Read the model definition and answer for the solid it produces. Units are mm, in the model's axes. A direction names the side the tool comes from. Give positions to 0.01 mm unless a question says otherwise; leave off trailing zeros. Write each loop counter-clockwise with the first axis right and the second up, starting at its lowest first coordinate (ties: lowest second). Pieces come first, ordered by that corner, then holes. Notation, with made-up numbers: M 63.25,-13 L 117.25,-13 A28 ccw 117.25,11 Z; hole C 72,28.5 d9. An arc over 180 degrees is marked long. Put each result on its own line as item: value.
from build123d import *

# Parameters (mm, degrees)
F6_R     = 3.175
F7_DEPTH = 177.8


with BuildPart() as f1:
    # F0 (on Front) → F1 (revolve)
    with BuildSketch(Plane.XZ):
        with BuildLine():
            Line((-134.874, 9.73), (-134.874, 0))
            Line((-134.874, 0), (134.874, 0))
            Line((134.874, 0), (134.874, 9.73))
            ThreePointArc((134.874, 9.73), (134.502026, 10.628026), (133.604, 11))
            Line((133.604, 11), (90.424, 11))
            Line((90.424, 11), (90.424, 13))
            Line((90.424, 13), (77.724, 13))
            Line((77.724, 13), (77.724, 32.05))
            Line((77.724, 32.05), (74.549, 32.05))
            Line((74.549, 32.05), (74.549, 13))
            Line((74.549, 13), (-74.549, 13))
            Line((-74.549, 13), (-74.549, 32.05))
            Line((-74.549, 32.05), (-77.724, 32.05))
            Line((-77.724, 32.05), (-77.724, 13))
            Line((-77.724, 13), (-90.424, 13))
            Line((-90.424, 13), (-90.424, 11))
            Line((-90.424, 11), (-133.604, 11))
            ThreePointArc((-133.604, 11), (-134.502026, 10.628026), (-134.874, 9.73))
        make_face()
    revolve(axis=Axis((-8.171387, 0, 0), (1, 0, 0)))


with BuildPart() as f2_1:
    # F2: copy of F1
    add(f1.part)


with BuildPart() as f4_1:
    # F4: copy of F2_1
    add(f2_1.part)

    # F6 (on face) → F7 (cut)
    with BuildSketch(Plane(origin=(-77.724, 0, 0), x_dir=(0, -1, 0), z_dir=(-1, 0, 0))):
        with Locations((0, 21.9075)):
            Circle(F6_R)
        with Locations((-21.9075, 0)):
            Circle(F6_R)
        with Locations((0, -21.9075)):
            Circle(F6_R)
        with Locations((21.9075, 0)):
            Circle(F6_R)
    extrude(amount=-F7_DEPTH, mode=Mode.SUBTRACT)


solid = f4_1.part
(1) Which of the six approach directions +Z, -Z, +X, -X, +Y, -Y give full straight-line access (tool end or side, diameter ignored) to faces 4 (the face through (90.424, -3, 11)), 5 (the face through (76.11, 25.08, 0.14)), 6 (the face through (-77.724, 0, 14)), 7 (the face through (-1.044, 7.91, -10.316))?
Result:
face 4: +X
face 5: +X, -X
face 6: -X
face 7: none
(2) Section C-C on x = 57.5 is taken. Determine the outline of the cut face in (y, z).
Result:
outline: C 0,0 d26
(3) Straight lines are drawn through the part: line 1 along Z through (x, y) = (75.6, 0); line 2 along X through (y, z) = (26, -3.5); line 3 along Y through (x, z) = (111.5, -1). For each, find the intervals that lie inside material, in ascending order. Write a range as from..to.
Result:
line 1: z = -32.05..-25.08, -18.73..18.73, 25.08..32.05
line 2: x = -77.72..-74.55, 74.55..77.72
line 3: y = -10.95..10.95
(4) For a pull along Y with two mould halves and no side action, classify faces 1 (the face through (76.114, -18.736, 0.14)), 2 (the face through (-134.874, 0, 0)), 3 (the face through (-112.32, 10.74, -2.38)) as +Y half, -Y half, draft (parallel to the pull), parting line (faces both ways), or undercut.
Result:
face 1: undercut
face 2: draft
face 3: parting line
(5) Section A-A on y = 0 is taken. Give the number of separate pieces and of enclosed holes in the cut face, and give its area (3 significant figures).
Result:
separate pieces: 5
enclosed holes: 0
area: 6,820 mm²
(6) Given pin 1 Ø8 at (x, y) = (98.5, -9.5) entering from -Z; pin 2 Ø5.5 at (y, z) = (0, -21.91) entering from -X; pin 3 Ø7.5 at (y, z) = (0, 21.91) entering from +X; pin 4 Ø12 at (y, z) = (5, -18) entering from +X, each flat-ended and moving along its own axis, determine where each tip first touches the part or whether it passes through.
Result:
pin 1: stops at z = -9.53
pin 2: passes through
pin 3: stops at x = 77.72
pin 4: stops at x = 90.42
